Work out the finished part from the listing and answer in its coordinate system (mm). Face numbers are marked on the shaded views. A direction names the side the tool comes from. Give positions to 0.01 mm unless a question says otherwise; leave off trailing zeros. Order: outer loops, then holes, each group sorted by start corner. A loop starts at its lowest first (then second) coordinate and runs counter-clockwise, first axis right, second up. Notation, with made-up numbers: (24.25, 27.5) - (67.25, 27.5) arc R18 ccw to (67.25, 42.5) - close; hole circle Ø6 at (79.25, 65). An arc over 180 degrees is marked (long way). Put each result on its own line as item: value.
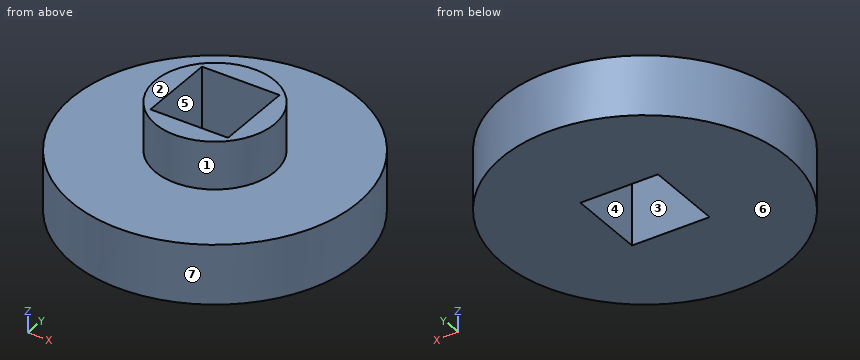
Autodesk Inventor part; units mm, degrees
ref_plane "YZ Plane" through (0, 0, 0) normal (1, 0, 0) x (0, 1, 0)
ref_plane "XZ Plane" through (0, 0, 0) normal (0, 1, 0) x (-1, 0, 0)
ref_plane "XY Plane" through (0, 0, 0) normal (0, 0, 1) x (1, 0, 0)
sketch "Sketch1" plane through (0, 0, 0) normal (0, 0, 1) x (1, 0, 0)
  circle A0 centre (0, 0) radius 12
  line L0 (-3.25, 3.25) -> (3.25, 3.25)
  line L1 (3.25, 3.25) -> (3.25, -3.25)
  line L2 (3.25, -3.25) -> (-3.25, -3.25)
  line L3 (-3.25, -3.25) -> (-3.25, 3.25)
  dimension "d0" = 24
  dimension "d1" = 6.5
extrude "Extrusion1" add sketch "Sketch1" along normal blind 5
sketch "Sketch2" plane through (0, 0, 5) normal (0, 0, 1) x (1, 0, 0)
  circle A0 centre (0, 0) radius 5
  line L0 (-3.25, 3.25) -> (3.25, 3.25)
  line L1 (3.25, 3.25) -> (3.25, -3.25)
  line L2 (3.25, -3.25) -> (-3.25, -3.25)
  line L3 (-3.25, -3.25) -> (-3.25, 3.25)
  line L4 (-3.25, 3.25) -> (3.25, 3.25)
  point P0 (0, 3.25)
extrude "Extrusion2" add sketch "Sketch2" along normal blind 4
properties part number "secondwheel"
(1) Determine the mould class of the marked faces 4, 5, 6 and 7 for opening direction Y: pulls with the +Y half, pulls with the -Y half, needs draft (parallel to the pull), parting line crosses it, or undercut.
Geometry check:
face 4: undercut
face 5: undercut
face 6: needs draft
face 7: parting line crosses it
(2) Straight lines are drawn through the part: line 1 (Z direction, x = -5.75, y = 9); line 2 (X direction, y = 1.5, z = 3.5); line 3 (Y direction, x = -0.75, z = 2.75). For each, find the intervals that lie inside material, in ascending order.
Geometry check:
line 1: z = 0 to 5
line 2: x = -11.91 to -3.25, 3.25 to 11.91
line 3: y = -11.98 to -3.25, 3.25 to 11.98
(3) Section C-C, the plane z = 0.75 is taken. Write down the section's boundary in (x, y), then the cut area to 3 significant figures.
Geometry check:
outline: circle Ø24 at (0, 0); hole (-3.25, -3.25) - (3.25, -3.25) - (3.25, 3.25) - (-3.25, 3.25) - close
area: 410 mm²
(4) Section D-D, the plane z = 7 is taken. Write down the section's boundary in (x, y), then the cut area to 3 significant figures.
Geometry check:
outline: circle Ø10 at (0, 0); hole (-3.25, -3.25) - (3.25, -3.25) - (3.25, 3.25) - (-3.25, 3.25) - close
area: 36.3 mm²
(5) Given pin 1 (2 mm diameter, centred on y = -0.5, z = 6.5, fed in from +X); pin 2 (1.5 mm diameter, centred on x = 3.5, z = 1, fed in from +Y); pin 3 (1.5 mm diameter, centred on x = -4.5, z = 5, fed in from +Y), each flat-ended and moving along its own axis, determine where each tip first touches the part or whether it passes through.
Geometry check:
pin 1: stops at x = 5
pin 2: stops at y = 11.68
pin 3: stops at y = 11.4
(6) Section A-A, the plane y = 0 is taken. Write down the section's boundary in (x, z), then the cut area to 4 significant figures.
Geometry check:
outline: (-12, 0) - (-3.25, 0) - (-3.25, 9) - (-5, 9) - (-5, 5) - (-12, 5) - close; (3.25, 0) - (12, 0) - (12, 5) - (5, 5) - (5, 9) - (3.25, 9) - close
area: 101.5 mm²
(7) A tool of negligible diameter and unlimited length cuts with its end or side. For the marked faces 1, 2 and 3, from which of +Z, -Z, +X, -X, +Y, -Y can it reach the whole face along a straight path? Write none if from no direction.
Geometry check:
face 1: +Z
face 2: +Z, +X, -X, +Y, -Y
face 3: +Z, -Z
